```python
from build123d import *

# Parameters (mm, degrees)
ESQUISSE1_W                            = 235
ESQUISSE1_H                            = 260
BOSS_EXTRU_1_DEPTH                     = 5
ENL_V_MAT_EXTRU_1_DEPTH                = 351.499643366
CHANFREIN1_SIZE                        = 20
CONG_1_R                               = 15
CHANFREIN2_SIZE                        = 20
CONG_2_R                               = 15
ENL_V_MAT_EXTRU_2_DEPTH                = 351.499643366
CHANFREIN3_SIZE                        = 20
CHANFREIN4_SIZE                        = 20
CONG_3_R                               = 15
BOSS_EXTRU_3_DEPTH                     = 5
TENON_ET_MORTAISE_TENON1_DEPTH         = 5
TENON_START                            = -260
TENON_ET_MORTAISE_RAINURE1_OUTLINE_W   = 15.2
TENON_ET_MORTAISE_RAINURE1_OUTLINE_H   = 5
TENON_ET_MORTAISE_RAINURE1_DEPTH       = 5.1
TENON_START_2                          = -208.886796564
TENON_ET_MORTAISE_RAINURE2_OUTLINE_W   = 4.9
TENON_ET_MORTAISE_RAINURE2_OUTLINE_H   = 5
TENON_ET_MORTAISE_RAINURE2_DEPTH       = 15.2
TENON_START_3                          = -184.947711832
TENON_ET_MORTAISE_RAINURE2_2_OUTLINE_W = 4.9
TENON_ET_MORTAISE_RAINURE2_2_OUTLINE_H = 5
TENON_ET_MORTAISE_RAINURE2_2_DEPTH     = 15.2
TENON_START_4                          = -161.008627099
TENON_ET_MORTAISE_RAINURE2_3_OUTLINE_W = 4.9
TENON_ET_MORTAISE_RAINURE2_3_OUTLINE_H = 5
TENON_ET_MORTAISE_RAINURE2_3_DEPTH     = 15.2
TENON_START_5                          = -137.069542366
TENON_ET_MORTAISE_RAINURE2_4_OUTLINE_W = 4.9
TENON_ET_MORTAISE_RAINURE2_4_OUTLINE_H = 5
TENON_ET_MORTAISE_RAINURE2_4_DEPTH     = 15.2
TENON_START_6                          = -113.130457634
TENON_ET_MORTAISE_RAINURE2_5_OUTLINE_W = 4.9
TENON_ET_MORTAISE_RAINURE2_5_OUTLINE_H = 5
TENON_ET_MORTAISE_RAINURE2_5_DEPTH     = 15.2
TENON_START_7                          = -89.191372901
TENON_ET_MORTAISE_RAINURE2_6_OUTLINE_W = 4.9
TENON_ET_MORTAISE_RAINURE2_6_OUTLINE_H = 5
TENON_ET_MORTAISE_RAINURE2_6_DEPTH     = 15.2
TENON_START_8                          = -65.252288168
TENON_ET_MORTAISE_RAINURE2_7_OUTLINE_W = 4.9
TENON_ET_MORTAISE_RAINURE2_7_OUTLINE_H = 5
TENON_ET_MORTAISE_RAINURE2_7_DEPTH     = 15.2
TENON_START_9                          = -41.313203436
TENON_ET_MORTAISE_RAINURE2_8_OUTLINE_W = 4.9
TENON_ET_MORTAISE_RAINURE2_8_OUTLINE_H = 5
TENON_ET_MORTAISE_RAINURE2_8_DEPTH     = 15.2
ESQUISSE6_R                            = 2.25
ENL_V_MAT_EXTRU_3_DEPTH                = 351.499643366


# Read off the part's stored shape, not the designer's step: Tenon et mortaise-Tenon1, Tenon et mortaise-Rainure1, Tenon et mortaise-Rainure2
with BuildPart() as part:
    # Esquisse1 → Boss.-Extru.1 (new body)
    with BuildSketch(Plane.XY):
        with Locations((-117.5, -130)):
            Rectangle(ESQUISSE1_W, ESQUISSE1_H)
    extrude(amount=BOSS_EXTRU_1_DEPTH)

    # Esquisse2 → Enlèv. mat.-Extru.1 (cut, through all)
    with BuildSketch(Plane.XY.offset(5)):
        with BuildLine():
            Line((-235, -88.457244293), (-235, -171.541538838))
            ThreePointArc((-235, -171.541538838), (-176.5, -129.999391565), (-235, -88.457244293))
        make_face()
    extrude(amount=-ENL_V_MAT_EXTRU_1_DEPTH, mode=Mode.SUBTRACT)

    # Chanfrein1
    chanfrein1_edges = [part.edges().sort_by_distance(p)[0] for p in [
        (-235, -260, 2.5),
    ]]
    chamfer(chanfrein1_edges, length=CHANFREIN1_SIZE)

    # Congé1
    cong_1_edges = [part.edges().sort_by_distance(p)[0] for p in [
        (-215, -260, 2.5),
        (-235, -240, 2.5),
    ]]
    fillet(cong_1_edges, radius=CONG_1_R)

    # Chanfrein2
    chanfrein2_edges = [part.edges().sort_by_distance(p)[0] for p in [
        (-235, 0, 2.5),
    ]]
    chamfer(chanfrein2_edges, length=CHANFREIN2_SIZE)

    # Congé2
    cong_2_edges = [part.edges().sort_by_distance(p)[0] for p in [
        (-235, -20, 2.5),
        (-215, 0, 2.5),
    ]]
    fillet(cong_2_edges, radius=CONG_2_R)

    # Esquisse4 → Enlèv. mat.-Extru.2 (cut, through all)
    with BuildSketch(Plane(origin=(0, 0, 0), x_dir=(-1, 0, 0), z_dir=(0, 0, -1))):
        with BuildLine():
            Line((20, -195), (160, -195))
            ThreePointArc((160, -195), (167.071067812, -192.071067812), (170, -185))
            Line((170, -185), (170, -105))
            ThreePointArc((170, -105), (167.071067812, -97.928932188), (160, -95))
            Line((160, -95), (60, -95))
            ThreePointArc((60, -95), (52.928932188, -97.928932188), (50, -105))
            Line((50, -105), (50, -135))
            ThreePointArc((50, -135), (47.071067812, -142.071067812), (40, -145))
            Line((40, -145), (20, -145))
            ThreePointArc((20, -145), (12.928932188, -147.928932188), (10, -155))
            Line((10, -155), (10, -185))
            ThreePointArc((10, -185), (12.928932188, -192.071067812), (20, -195))
        make_face()
    extrude(amount=-ENL_V_MAT_EXTRU_2_DEPTH, mode=Mode.SUBTRACT)

    # Chanfrein3
    chanfrein3_edges = [part.edges().sort_by_distance(p)[0] for p in [
        (0, -260, 2.5),
    ]]
    chamfer(chanfrein3_edges, length=CHANFREIN3_SIZE)

    # Chanfrein4
    chanfrein4_edges = [part.edges().sort_by_distance(p)[0] for p in [
        (0, 0, 2.5),
    ]]
    chamfer(chanfrein4_edges, length=CHANFREIN4_SIZE)

    # Congé3
    cong_3_edges = [part.edges().sort_by_distance(p)[0] for p in [
        (0, -240, 2.5),
        (-20, -260, 2.5),
        (-20, 0, 2.5),
        (0, -20, 2.5),
        (-235, -171.541538838, 2.5),
        (-235, -88.457244293, 2.5),
    ]]
    fillet(cong_3_edges, radius=CONG_3_R)

    # Esquisse5 → Boss.-Extru.3 (add, through all)
    with BuildSketch(Plane(origin=(0, 0, 0), x_dir=(-1, 0, 0), z_dir=(0, 0, -1))):
        with BuildLine():
            ThreePointArc((117, -195), (109.928932188, -192.071067812), (107, -185))
            Line((107, -185), (107, -105))
            ThreePointArc((107, -105), (109.928932188, -97.928932188), (117, -95))
            Line((117, -95), (60, -95))
            ThreePointArc((60, -95), (52.928932188, -97.928932188), (50, -105))
            Line((50, -105), (50, -135))
            ThreePointArc((50, -135), (47.071067812, -142.071067812), (40, -145))
            Line((40, -145), (20, -145))
            ThreePointArc((20, -145), (12.928932188, -147.928932188), (10, -155))
            Line((10, -155), (10, -185))
            ThreePointArc((10, -185), (12.928932188, -192.071067812), (20, -195))
            Line((20, -195), (117, -195))
        make_face()
    extrude(amount=-BOSS_EXTRU_3_DEPTH)

    # Tenon et mortaise-Tenon1 outline → Tenon et mortaise-Tenon1 (add)
    with BuildSketch(Plane.XY):
        Polygon((0, -26.213203436), (0, -41.213203436), (4, -41.213203436), (5, -40.213203436), (5, -27.213203436), (4, -26.213203436), align=None)
        Polygon((0, -53.72371674), (0, -68.72371674), (4, -68.72371674), (5, -67.72371674), (5, -54.72371674), (4, -53.72371674), align=None)
        Polygon((0, -81.234230044), (0, -96.234230044), (4, -96.234230044), (5, -95.234230044), (5, -82.234230044), (4, -81.234230044), align=None)
        Polygon((0, -108.744743348), (0, -123.744743348), (4, -123.744743348), (5, -122.744743348), (5, -109.744743348), (4, -108.744743348), align=None)
        Polygon((0, -136.255256652), (0, -151.255256652), (4, -151.255256652), (5, -150.255256652), (5, -137.255256652), (4, -136.255256652), align=None)
        Polygon((0, -163.765769956), (0, -178.765769956), (4, -178.765769956), (5, -177.765769956), (5, -164.765769956), (4, -163.765769956), align=None)
        Polygon((0, -191.27628326), (0, -206.27628326), (4, -206.27628326), (5, -205.27628326), (5, -192.27628326), (4, -191.27628326), align=None)
        Polygon((4, -218.786796564), (0, -218.786796564), (0, -233.786796564), (4, -233.786796564), (5, -232.786796564), (5, -219.786796564), align=None)
    extrude(amount=TENON_ET_MORTAISE_TENON1_DEPTH)

    # Tenon et mortaise-Rainure1 outline → Tenon et mortaise-Rainure1 (cut)
    with BuildSketch(Plane(origin=(0, 0, 0), x_dir=(1, 0, 0), z_dir=(0, 1, 0)).offset(TENON_START)):
        with Locations((-33.713203436, -2.5)):
            Rectangle(TENON_ET_MORTAISE_RAINURE1_OUTLINE_W, TENON_ET_MORTAISE_RAINURE1_OUTLINE_H)
        with Locations((-57.652288168, -2.5)):
            Rectangle(TENON_ET_MORTAISE_RAINURE1_OUTLINE_W, TENON_ET_MORTAISE_RAINURE1_OUTLINE_H)
        with Locations((-81.591372901, -2.5)):
            Rectangle(TENON_ET_MORTAISE_RAINURE1_OUTLINE_W, TENON_ET_MORTAISE_RAINURE1_OUTLINE_H)
        with Locations((-105.530457634, -2.5)):
            Rectangle(TENON_ET_MORTAISE_RAINURE1_OUTLINE_W, TENON_ET_MORTAISE_RAINURE1_OUTLINE_H)
        with Locations((-129.469542366, -2.5)):
            Rectangle(TENON_ET_MORTAISE_RAINURE1_OUTLINE_W, TENON_ET_MORTAISE_RAINURE1_OUTLINE_H)
        with Locations((-153.408627099, -2.5)):
            Rectangle(TENON_ET_MORTAISE_RAINURE1_OUTLINE_W, TENON_ET_MORTAISE_RAINURE1_OUTLINE_H)
        with Locations((-177.347711832, -2.5)):
            Rectangle(TENON_ET_MORTAISE_RAINURE1_OUTLINE_W, TENON_ET_MORTAISE_RAINURE1_OUTLINE_H)
        with Locations((-201.286796564, -2.5)):
            Rectangle(TENON_ET_MORTAISE_RAINURE1_OUTLINE_W, TENON_ET_MORTAISE_RAINURE1_OUTLINE_H)
    extrude(amount=TENON_ET_MORTAISE_RAINURE1_DEPTH, mode=Mode.SUBTRACT)

    # Tenon et mortaise-Rainure2 outline → Tenon et mortaise-Rainure2 (cut)
    with BuildSketch(Plane.YZ.offset(TENON_START_2)):
        with Locations((-2.45, 2.5)):
            Rectangle(TENON_ET_MORTAISE_RAINURE2_OUTLINE_W, TENON_ET_MORTAISE_RAINURE2_OUTLINE_H)
    extrude(amount=TENON_ET_MORTAISE_RAINURE2_DEPTH, mode=Mode.SUBTRACT)

    # Tenon et mortaise-Rainure2 2 outline → Tenon et mortaise-Rainure2 2 (cut)
    with BuildSketch(Plane.YZ.offset(TENON_START_3)):
        with Locations((-2.45, 2.5)):
            Rectangle(TENON_ET_MORTAISE_RAINURE2_2_OUTLINE_W, TENON_ET_MORTAISE_RAINURE2_2_OUTLINE_H)
    extrude(amount=TENON_ET_MORTAISE_RAINURE2_2_DEPTH, mode=Mode.SUBTRACT)

    # Tenon et mortaise-Rainure2 3 outline → Tenon et mortaise-Rainure2 3 (cut)
    with BuildSketch(Plane.YZ.offset(TENON_START_4)):
        with Locations((-2.45, 2.5)):
            Rectangle(TENON_ET_MORTAISE_RAINURE2_3_OUTLINE_W, TENON_ET_MORTAISE_RAINURE2_3_OUTLINE_H)
    extrude(amount=TENON_ET_MORTAISE_RAINURE2_3_DEPTH, mode=Mode.SUBTRACT)

    # Tenon et mortaise-Rainure2 4 outline → Tenon et mortaise-Rainure2 4 (cut)
    with BuildSketch(Plane.YZ.offset(TENON_START_5)):
        with Locations((-2.45, 2.5)):
            Rectangle(TENON_ET_MORTAISE_RAINURE2_4_OUTLINE_W, TENON_ET_MORTAISE_RAINURE2_4_OUTLINE_H)
    extrude(amount=TENON_ET_MORTAISE_RAINURE2_4_DEPTH, mode=Mode.SUBTRACT)

    # Tenon et mortaise-Rainure2 5 outline → Tenon et mortaise-Rainure2 5 (cut)
    with BuildSketch(Plane.YZ.offset(TENON_START_6)):
        with Locations((-2.45, 2.5)):
            Rectangle(TENON_ET_MORTAISE_RAINURE2_5_OUTLINE_W, TENON_ET_MORTAISE_RAINURE2_5_OUTLINE_H)
    extrude(amount=TENON_ET_MORTAISE_RAINURE2_5_DEPTH, mode=Mode.SUBTRACT)

    # Tenon et mortaise-Rainure2 6 outline → Tenon et mortaise-Rainure2 6 (cut)
    with BuildSketch(Plane.YZ.offset(TENON_START_7)):
        with Locations((-2.45, 2.5)):
            Rectangle(TENON_ET_MORTAISE_RAINURE2_6_OUTLINE_W, TENON_ET_MORTAISE_RAINURE2_6_OUTLINE_H)
    extrude(amount=TENON_ET_MORTAISE_RAINURE2_6_DEPTH, mode=Mode.SUBTRACT)

    # Tenon et mortaise-Rainure2 7 outline → Tenon et mortaise-Rainure2 7 (cut)
    with BuildSketch(Plane.YZ.offset(TENON_START_8)):
        with Locations((-2.45, 2.5)):
            Rectangle(TENON_ET_MORTAISE_RAINURE2_7_OUTLINE_W, TENON_ET_MORTAISE_RAINURE2_7_OUTLINE_H)
    extrude(amount=TENON_ET_MORTAISE_RAINURE2_7_DEPTH, mode=Mode.SUBTRACT)

    # Tenon et mortaise-Rainure2 8 outline → Tenon et mortaise-Rainure2 8 (cut)
    with BuildSketch(Plane.YZ.offset(TENON_START_9)):
        with Locations((-2.45, 2.5)):
            Rectangle(TENON_ET_MORTAISE_RAINURE2_8_OUTLINE_W, TENON_ET_MORTAISE_RAINURE2_8_OUTLINE_H)
    extrude(amount=TENON_ET_MORTAISE_RAINURE2_8_DEPTH, mode=Mode.SUBTRACT)

    # Esquisse6 → Enlèv. mat.-Extru.3 (cut, through all)
    with BuildSketch(Plane.XY.offset(5)):
        with Locations((-209.25, -43.5)):
            Circle(ESQUISSE6_R)
        with Locations((-219.25, -43.5)):
            Circle(ESQUISSE6_R)
    enl_v_mat_extru_3 = extrude(amount=-ENL_V_MAT_EXTRU_3_DEPTH, mode=Mode.SUBTRACT)

    # Symétrie1: Enlèv. mat.-Extru.3 across plane
    add(enl_v_mat_extru_3.mirror(Plane.ZX.offset(-130)), mode=Mode.SUBTRACT)


solid = part.part
```
Can you work these out from the model? Positions are in its coordinate system, mm. A direction names the side the tool comes from. Round coordinates to 2 decimals unless told otherwise and drop trailing zeros. Order: outer loops, then holes, each group sorted by start corner. A loop starts at its lowest first (then second) coordinate and runs counter-clockwise, first axis right, second up. Notation, with made-up numbers: (-36.5, 19) -> (13.5, 19) arc R24 ccw to (13.5, 53) -> close; hole circle Ø11 at (-11.5, -31). An arc over 180 degrees is marked (long way). Return JSON: item names as keys, results as strings. Group by question number.
1. Will these pins go through, and if not, where does the flat tip stop? pin 1 (1.5 mm diameter, centred on y = -130, z = 2.5, fed in from +X); pin 2 (3 mm diameter, centred on x = 2.5, z = 1.5, fed in from -Y); pin 3 (1.5 mm diameter, centred on y = -2.5, z = 2.5, fed in from -X).
2. I need wall thicknesses on line 1 (X direction, y = -216.5, z = 1.2); line 2 (X direction, y = -217, z = 3.3); line 3 (Y direction, x = -209, z = 0.6). Which ranges of each line are inside material? Lowest first, please. Write a range as [from, to].
3. If we section it at B-B, the plane x = -181: Write out the boundary of the cut face in (y, z), then the cut area to 3 significant figures.
4. If we section it at C-C, the plane z = 0.9: Count the separate pieces of the cut face and the enclosed holes in it, then the cut area to 3 significant figures.
5. If we section it at D-D, the plane x = -18.5: Write out the boundary of the cut face in (y, z).
6. If we section it at A-A, the plane y = -147: Write out the boundary of the cut face in (x, z).
7. We'd pull the mould along X, two halves only. Please class faces 4 (the face through (-10, -250, 2)), 5 (the face through (-225, -250, 2)), 6 (the face through (-167.15, -98.01, 2.46)): released by +X, released by -X, zero draft, split by the parting line, or undercut.
8. Which directions (+Z, -Z, +X, -X, +Y, -Y) give clear straight access to the entire face, cutting with the end or side of a thin tool? Please do faces 1 (the face through (-10, -10, 2)), 2 (the face through (-109.85, -98.01, 2.46)), 3 (the face through (-230.766, -178.553, 2.465)).
Output values:
{
 "1": {"pin 1": "x = 0", "pin 2": "y = -233.79", "pin 3": "x = -218.11"},
 "2": {"line 1": "[-235, -221.5], [-217, -211.5], [-207, 0]", "line 2": "[-235, -221.44], [-217.06, -211.44], [-207.06, 0]", "line 3": "[-260, -218.74], [-214.26, -172.47], [-87.53, -45.74], [-41.26, 0]"},
 "3": {"outline": "(-254.9, 0) -> (-149.38, 0) -> (-149.38, 5) -> (-254.9, 5) -> close; (-110.62, 0) -> (-4.9, 0) -> (-4.9, 5) -> (-110.62, 5) -> close", "area": "1,060 mm²"},
 "4": {"separate pieces": "1", "enclosed holes": "5", "area": "48,900 mm²"},
 "5": {"outline": "(-257.86, 0) -> (-2.14, 0) -> (-2.14, 5) -> (-257.86, 5) -> close"},
 "6": {"outline": "(-179.92, 0) -> (-170, 0) -> (-170, 5) -> (-179.92, 5) -> close; (-107, 0) -> (5, 0) -> (5, 5) -> (-107, 5) -> close"},
 "7": {"face 4": "released by +X", "face 5": "released by -X", "face 6": "undercut"},
 "8": {"face 1": "+Z, -Z, +X, +Y", "face 2": "+Z, -Z", "face 3": "+Z, -Z, -X"}
}
